The listing builds one solid part. Answer for the finished solid, in the listing's coordinates (mm). Face numbers are marked on the shaded views. A direction names the side the tool comes from. Give positions to 0.01 mm unless a question says otherwise; leave off trailing zeros. Order: outer loops, then holes, each group sorted by start corner. A loop starts at its lowest first (then second) coordinate and runs counter-clockwise, first axis right, second up. Notation, with made-up numbers: (79.25, 22.5) - (98.25, 22.5) arc R12 cw to (98.25, 44.5) - close; hole circle Ø5 at (-28.75, 21.5). An arc over 180 degrees is marked (long way). Write each question's results on one line, items separated by ' | '. Start each with the question number.
1. Section D-D (z = 3) is taken. Give the vertices of the cut face in (x, y), and give its area (3 significant figures).
2. Section C-C (x = 6.25) is taken. Give the vertices of the cut face in (y, z), and give its area (3 significant figures).
3. Flat-ended cylindrical pins translate along their axes: pin 1 (0.8 mm diameter, centred on x = 3, y = -2.5, fed in from -Z); pin 2 (0.8 mm diameter, centred on y = -3, z = 0.5, fed in from +X) (3 decimals); pin 3 (1.5 mm diameter, centred on y = -3, z = 4.5, fed in from -X). Find the tip coordinate at first contact, or state that the pin passes through.
4. Which of the six approach directions +Z, -Z, +X, -X, +Y, -Y give full straight-line access (tool end or side, diameter ignored) to the marked faces 1 and 2?
5. Find the intervals of material crossed by L1, parallel to Z at x = 9, y = -2.5; L2, parallel to Z at x = 2.75, y = -1.4; L3, parallel to X at y = -2.4, z = 3.75, in increasing order.
6. Section B-B (y = -1.85) is taken. Give the vertices of the cut face in (x, z).
7. Section A-A (z = 0.5) is taken. Give the vertices of the cut face in (x, y), and give its area (3 significant figures).
8. Determine the mould class of the marked faces 3, 4 and 5 for opening direction Y: released by +Y, released by -Y, zero draft, split by the parting line, or undercut.
from build123d import *

# Parameters (mm, degrees)
F1_DEPTH = 1.5
F2_R     = 1.75
F3_DEPTH = 5
F4_W     = 2.7
F4_H     = 2.7
F5_DEPTH = 1


with BuildPart() as f1:
    # F0 (on Top) → F1 (new body)
    with BuildSketch(Plane.XY):
        with BuildLine():
            Line((-0.651671, -4.7), (-0.651671, 0))
            ThreePointArc((-0.651671, 0), (-3.001671, -2.35), (-0.651671, -4.7))
        make_face()
        with BuildLine():
            ThreePointArc((1.698329, -2.35), (1.01003, -0.688299), (-0.651671, 0))
            Line((-0.651671, 0), (-0.651671, -4.7))
            ThreePointArc((-0.651671, -4.7), (1.01003, -4.011701), (1.698329, -2.35))
        make_face()
        with BuildLine():
            Line((7.648329, 0), (-0.651671, 0))
            ThreePointArc((-0.651671, 0), (1.01003, -0.688299), (1.698329, -2.35))
            ThreePointArc((1.698329, -2.35), (1.01003, -4.011701), (-0.651671, -4.7))
            Line((-0.651671, -4.7), (7.648329, -4.7))
            ThreePointArc((7.648329, -4.7), (5.298329, -2.35), (7.648329, 0))
        make_face()
        with BuildLine():
            ThreePointArc((9.998329, -2.35), (9.31003, -0.688299), (7.648329, 0))
            Line((7.648329, 0), (7.648329, -4.7))
            ThreePointArc((7.648329, -4.7), (9.31003, -4.011701), (9.998329, -2.35))
        make_face()
        with BuildLine():
            Line((7.648329, -4.7), (7.648329, 0))
            ThreePointArc((7.648329, 0), (5.298329, -2.35), (7.648329, -4.7))
        make_face()
    extrude(amount=F1_DEPTH)

    # F2 (on face) → F3 (join)
    with BuildSketch(Plane.XY.offset(1.5)):
        with Locations((3.498329, -2.35)):
            Circle(F2_R)
    extrude(amount=F3_DEPTH)

    # F4 (on face) → F5 (cut)
    with BuildSketch(Plane(origin=(0, 0, 0), x_dir=(1, 0, 0), z_dir=(0, 0, -1))):
        with Locations((3.498329, 2.35)):
            Rectangle(F4_W, F4_H)
    extrude(amount=-F5_DEPTH, mode=Mode.SUBTRACT)


solid = f1.part
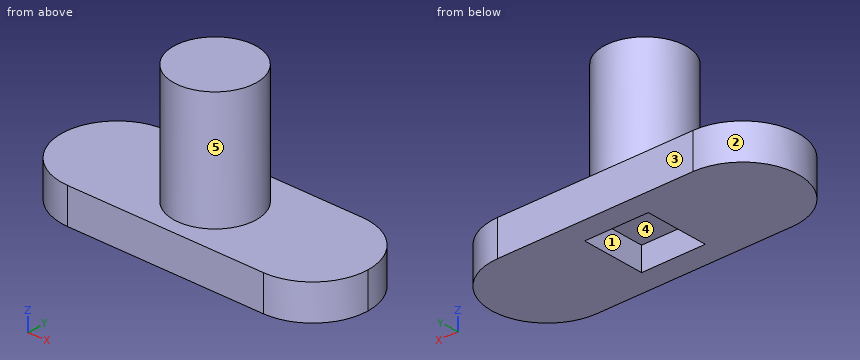
Reported:
1) outline: circle Ø3.5 at (3.5, -2.35) | area: 9.62 mm²
2) outline: (-4.7, 0) - (0, 0) - (0, 1.5) - (-4.7, 1.5) - close | area: 7.05 mm²
3) pin 1: z = 1 | pin 2: x = 9.985 | pin 3: x = 1.75
4) face 1: -Z | face 2: +Z, -Z, -X
5) L1: 0 to 1.5 | L2: 1 to 6.5 | L3: 1.75 to 5.25
6) outline: (-2.95, 0) - (2.15, 0) - (2.15, 1) - (4.85, 1) - (4.85, 0) - (9.94, 0) - (9.94, 1.5) - (5.18, 1.5) - (5.18, 6.5) - (1.82, 6.5) - (1.82, 1.5) - (-2.95, 1.5) - close
7) outline: (-0.65, -4.7) - (7.65, -4.7) arc R2.35 ccw to (7.65, 0) - (-0.65, 0) arc R2.35 ccw to start; hole (2.15, -3.7) - (4.85, -3.7) - (4.85, -1) - (2.15, -1) - close | area: 49.1 mm²
8) face 3: released by +Y | face 4: undercut | face 5: split by the parting line
